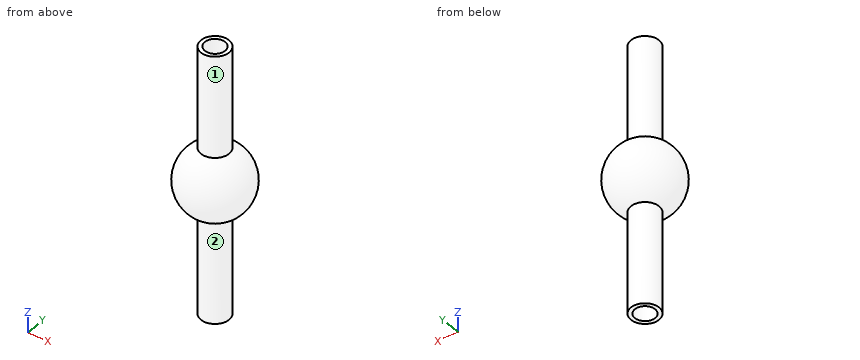
from build123d import *

# Parameters (mm, degrees)
CUT_EXTRUDE1_DEPTH       = 10
CUT_EXTRUDE1_DEPTH_BACK  = 10
SKETCH2_R                = 3.175
BOSS_EXTRUDE1_DEPTH      = 30
BOSS_EXTRUDE1_DEPTH_BACK = 30
SKETCH3_R                = 3.175
SKETCH3_R_2              = 2.286


with BuildPart() as part:
    # Sketch1 → Revolve1 (revolve)
    with BuildSketch(Plane(origin=(0, 0, 0), x_dir=(1, 0, 0), z_dir=(0, 1, 0))):
        with BuildLine():
            Line((0, 7.935), (0, -7.935))
            ThreePointArc((0, -7.935), (-7.935, 0), (0, 7.935))
        make_face()
    revolve(axis=Axis((0, 0, -16.813567773), (0, 0, 1)))

    # Sketch2 → Cut-Extrude1 (cut, two sides: drawn at the far end of the back side and taken through both)
    with BuildSketch(Plane.XY.offset(-CUT_EXTRUDE1_DEPTH_BACK)):
        with Locations(Location((0, 0, 0), (0, 0, 180))):
            Circle(SKETCH2_R)
    extrude(amount=CUT_EXTRUDE1_DEPTH + CUT_EXTRUDE1_DEPTH_BACK, mode=Mode.SUBTRACT)

    # Sketch3 → Boss-Extrude1 (add, two sides: drawn at the far end of the back side and taken through both)
    with BuildSketch(Plane.XY.offset(-BOSS_EXTRUDE1_DEPTH_BACK)):
        Circle(SKETCH3_R)
        Circle(SKETCH3_R_2, mode=Mode.SUBTRACT)
    extrude(amount=BOSS_EXTRUDE1_DEPTH + BOSS_EXTRUDE1_DEPTH_BACK)


solid = part.part
For this review, take the finished solid that the model builds, in its own axes (mm). Face numbers are marked on the shaded views. A direction names the side the tool comes from. Round coordinates to 2 decimals unless told otherwise and drop trailing zeros. Write each loop counter-clockwise with the first axis right and the second up, starting at its lowest first coordinate (ties: lowest second). Pieces come first, ordered by that corner, then holes. Notation, with made-up numbers: (56.25, -24) -> (75.25, -24) arc R18 ccw to (75.25, -14) -> close; hole circle Ø6 at (78, -23.5). An arc over 180 degrees is marked (long way). Use CSV: the item, a comma, the result in double quotes.
(1) Clearance check with flat-ended pins moving along their axes: P1, Ø1, axis at x = 4.5, y = -3.5, coming from the -Z side; P2, Ø8, axis at y = 2.5, z = 8, coming from the -X side; P3, Ø4, axis at x = -5, y = -6, coming from the -Z side. State where each tip first meets the part, or that it passes through.
Computed values:
P1,"z = -5.99"
P2,"x = -6.62"
P3,"z = -5.4"
(2) For the marked faces 1 and 2, list the 3-axis set-ups (+Z, -Z, +X, -X, +Y, -Y) from which the entire face can be reached by the end or side of a thin tool; tool diameter is ignored.
Computed values:
face 1,"+Z"
face 2,"-Z"
(3) Consider section D-D, the plane y = -6.75. Give the boundary of the cut face in (x, z), plus the area to 3 significant figures.
Computed values:
outline,"circle Ø8.34 at (0, 0)"
area,"54.7 mm²"
(4) Consider section C-C, the plane z = 20. Give the boundary of the cut face in (x, y) (3 decimals).
Computed values:
outline,"circle Ø6.35 at (0, 0); hole circle Ø4.572 at (0, 0)"
(5) To check wall thickness, follow L1, parallel to Y at x = 0, z = 15.5 (3 decimals); L2, parallel to X at y = 2, z = -2.5; L3, parallel to Y at x = 1.75, z = 23. State the ranges of each line that lie inside material, in increasing order. Write a range as [from, to].
Computed values:
L1,"[-3.175, -2.286], [2.286, 3.175]"
L2,"[-7.26, -1.11], [1.11, 7.26]"
L3,"[-2.65, -1.47], [1.47, 2.65]"
(6) Consider section A-A, the plane x = 0. Give the boundary of the cut face in (y, z) (3 decimals), plus the area to 3 significant figures.
Computed values:
outline,"(-3.175, -30) -> (-2.286, -30) -> (-2.286, 30) -> (-3.175, 30) -> (-3.175, 7.272) arc R7.935 ccw to (-3.175, -7.272) -> close; (2.286, -30) -> (3.175, -30) -> (3.175, -7.272) arc R7.935 ccw to (3.175, 7.272) -> (3.175, 30) -> (2.286, 30) -> close"
area,"206 mm²"
